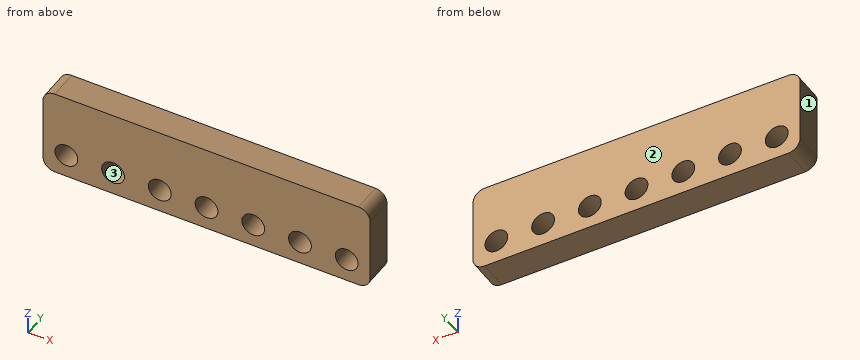
```python
from build123d import *

# Parameters (mm, degrees)
BOSS_EXTRUDE1_DEPTH = 5
SKETCH2_R           = 1.95
CUT_EXTRUDE1_DEPTH  = 6


with BuildPart() as part:
    # Sketch1 → Boss-Extrude1 (new body)
    with BuildSketch(Plane(origin=(0, 0, 0), x_dir=(1, 0, 0), z_dir=(0, 1, 0))):
        with BuildLine():
            Line((-54, 0), (-2, 0))
            ThreePointArc((-2, 0), (-0.585786438, -0.585786438), (0, -2))
            Line((0, -2), (0, -13))
            ThreePointArc((0, -13), (-0.585786438, -14.414213562), (-2, -15))
            Line((-2, -15), (-54, -15))
            ThreePointArc((-54, -15), (-55.414213562, -14.414213562), (-56, -13))
            Line((-56, -13), (-56, -2))
            ThreePointArc((-56, -2), (-55.414213562, -0.585786438), (-54, 0))
        make_face()
    extrude(amount=BOSS_EXTRUDE1_DEPTH)

    # Sketch2 → Cut-Extrude1 (cut, through all)
    with BuildSketch(Plane(origin=(0, 5, 0), x_dir=(1, 0, 0), z_dir=(0, 1, 0))):
        with Locations((-4, -4)):
            Circle(SKETCH2_R)
        with Locations((-12, -4)):
            Circle(SKETCH2_R)
        with Locations((-76, -4)):
            Circle(SKETCH2_R)
        with Locations((-68, -4)):
            Circle(SKETCH2_R)
        with Locations((-60, -4)):
            Circle(SKETCH2_R)
        with Locations((-52, -4)):
            Circle(SKETCH2_R)
        with Locations((-44, -4)):
            Circle(SKETCH2_R)
        with Locations((-36, -4)):
            Circle(SKETCH2_R)
        with Locations((-28, -4)):
            Circle(SKETCH2_R)
        with Locations((-20, -4)):
            Circle(SKETCH2_R)
    extrude(amount=-CUT_EXTRUDE1_DEPTH, mode=Mode.SUBTRACT)


solid = part.part
```
CAD build for the part. Positions are in the model's coordinates, mm. Face numbers are marked on the shaded views. Coordinates: 2 decimals unless noted, no trailing zeros. Order: outer loops, then holes, each group sorted by start corner. A loop starts at its lowest first (then second) coordinate and runs counter-clockwise, first axis right, second up. Notation, with made-up numbers: (62.25, -36) - (91.25, -36) arc R23 cw to (91.25, 0) - close; hole circle Ø5 at (25.25, -31.5). An arc over 180 degrees is marked (long way). Answer in a Markdown table with one row per item.
1. Drill centre lines: L1, parallel to Z at x = -12, y = 2.1; L2, parallel to X at y = 2.55, z = 1; L3, parallel to X at y = 2.55, z = 14.75. Where is each one in solid material? Low to high. Write a range as from..to.
Answer:
| item | result |
|---|---|
| L1 | 0..2.05, 5.95..15 |
| L2 | -55.73..-0.27 |
| L3 | -54.97..-1.03 |
2. Slice it at A-A, the plane x = -28. List the corners of the cut face in (y, z), then the cut area to 3 significant figures.
Answer:
| item | result |
|---|---|
| outline | (0, 0) - (5, 0) - (5, 2.05) - (0, 2.05) - close; (0, 5.95) - (5, 5.95) - (5, 15) - (0, 15) - close |
| area | 55.5 mm² |
3. Slice it at B-B, the plane y = 3.75. List the corners of the cut face in (x, z), then the cut area to 3 significant figures.
Answer:
| item | result |
|---|---|
| outline | (-56, 2) arc R2 ccw to (-54, 0) - (-2, 0) arc R2 ccw to (0, 2) - (0, 13) arc R2 ccw to (-2, 15) - (-54, 15) arc R2 ccw to (-56, 13) - close; hole circle Ø3.9 at (-52, 4); hole circle Ø3.9 at (-44, 4); hole circle Ø3.9 at (-36, 4); hole circle Ø3.9 at (-28, 4); hole circle Ø3.9 at (-20, 4); hole circle Ø3.9 at (-12, 4); hole circle Ø3.9 at (-4, 4) |
| area | 753 mm² |
4. Slice it at C-C, the plane z = 4. Give the number of separate pieces and of enclosed holes in the cut face, then the cut area to 4 significant figures.
Answer:
| item | result |
|---|---|
| separate pieces | 8 |
| enclosed holes | 0 |
| area | 143.5 mm² |
5. Slice it at D-D, the plane x = -37. List the corners of the cut face in (y, z), then the cut area to 3 significant figures.
Answer:
| item | result |
|---|---|
| outline | (0, 0) - (5, 0) - (5, 2.33) - (0, 2.33) - close; (0, 5.67) - (5, 5.67) - (5, 15) - (0, 15) - close |
| area | 58.3 mm² |
6. Pull direction X, two halves, no side cores. Call the marked faces 1, 2 and 3: +X half, -X half, draft (parallel to the pull), parting line (faces both ways), or undercut.
Answer:
| item | result |
|---|---|
| face 1 | -X half |
| face 2 | draft |
| face 3 | undercut |
